Read the model definition and answer for the solid it produces. Units are mm, in the model's axes. Face numbers are marked on the shaded views. A direction names the side the tool comes from. Coordinates: 2 decimals unless noted, no trailing zeros. Order: outer loops, then holes, each group sorted by start corner. A loop starts at its lowest first (then second) coordinate and runs counter-clockwise, first axis right, second up. Notation, with made-up numbers: (-12, 9.5) -> (-8, 9.5) arc R24 ccw to (-8, 35.5) -> close; hole circle Ø10 at (-31.5, 14). An arc over 180 degrees is marked (long way). Use CSV: the item, a comma, the result in double quotes.
```python
from build123d import *

# Parameters (mm, degrees)
F1_DEPTH = 25.4
F2_DEPTH = 25.654


with BuildPart() as f1:
    # F0 (on Front) → F1 (new body)
    with BuildSketch(Plane.XZ):
        with BuildLine():
            ThreePointArc((-15.060614174, 41.9682624685), (-0.0688082783, 50.3511332937), (14.987647146, 42.0849420703))
            ThreePointArc((14.987647146, 42.0849420703), (19.3434405932, 43.5057594661), (23.8204686342, 44.4793500101))
            Line((23.8204686342, 44.4793500101), (1.0321482392, 85.7816260454))
            Line((1.0321482392, 85.7816260454), (-24.0085215463, 44.2917114126))
            ThreePointArc((-24.0085215463, 44.2917114126), (-19.4747765312, 43.3602512097), (-15.060614174, 41.9682624685))
        make_face()
    extrude(amount=-F1_DEPTH)

    # F0 (on Front) → F2 (join)
    with BuildSketch(Plane.XZ):
        with BuildLine():
            Line((-28.8295803882, 36.30369346), (-27.7535005612, 38.0866513657))
            Line((-27.7535005612, 38.0866513657), (-30.7906209519, 44.8054462665))
            ThreePointArc((-30.7906209519, 44.8054462665), (-29.6489661187, 40.624103652), (-29.2771657497, 36.3056819144))
            Line((-29.2771657497, 36.3056819144), (-28.8295803882, 36.30369346))
        make_face()
        Polygon((-30.7906209519, 44.8054462665), (-27.7535005612, 38.0866513657), (-25.0648295944, 42.54151339), align=None)
        with BuildLine():
            Line((-53.3023555948, 36.4124168488), (-30.7906209519, 36.3124056299))
            Line((-30.7906209519, 36.3124056299), (-30.7906209519, 44.8054462665))
            ThreePointArc((-30.7906209519, 44.8054462665), (-62.5500321621, 31.6953988364), (-75.8140902377, 0))
            Line((-75.8140902377, 0), (-75.2328084137, -0.0011871857))
            ThreePointArc((-75.2328084137, -0.0011871857), (-73.1076200485, 9.3092127471), (-67.2269157832, 16.8336588954))
            ThreePointArc((-67.2269157832, 16.8336588954), (-60.6978163865, 20.5368755433), (-53.3023555948, 21.8214424558))
            Line((-53.3023555948, 21.8214424558), (-53.3023555948, 36.4124168488))
        make_face()
        with BuildLine():
            Line((-30.7906209519, 44.8054462665), (-30.7906209519, 36.3124056299))
            Line((-30.7906209519, 36.3124056299), (-29.2771657497, 36.3056819144))
            ThreePointArc((-29.2771657497, 36.3056819144), (-29.6489661187, 40.624103652), (-30.7906209519, 44.8054462665))
        make_face()
        with BuildLine():
            Line((-25.0648295944, 42.54151339), (-16.4788366985, 39.1466793172))
            ThreePointArc((-16.4788366985, 39.1466793172), (-15.832705808, 40.5891269445), (-15.060614174, 41.9682624685))
            ThreePointArc((-15.060614174, 41.9682624685), (-19.4747765312, 43.3602512097), (-24.0085215463, 44.2917114126))
            Line((-24.0085215463, 44.2917114126), (-25.0648295944, 42.54151339))
        make_face()
        with BuildLine():
            ThreePointArc((23.8204686342, 44.4793500101), (19.3434405932, 43.5057594661), (14.987647146, 42.0849420703))
            ThreePointArc((14.987647146, 42.0849420703), (15.7885662341, 40.6763432088), (16.4574657961, 39.2004721052))
            Line((16.4574657961, 39.2004721052), (24.8784135948, 42.5618969449))
            Line((24.8784135948, 42.5618969449), (23.8204686342, 44.4793500101))
        make_face()
        with BuildLine():
            ThreePointArc((-15.060614174, 41.9682624685), (-0.0688082783, 50.3511332937), (14.987647146, 42.0849420703))
            ThreePointArc((14.987647146, 42.0849420703), (19.3434405932, 43.5057594661), (23.8204686342, 44.4793500101))
            Line((23.8204686342, 44.4793500101), (1.0321482392, 85.7816260454))
            Line((1.0321482392, 85.7816260454), (-24.0085215463, 44.2917114126))
            ThreePointArc((-24.0085215463, 44.2917114126), (-19.4747765312, 43.3602512097), (-15.060614174, 41.9682624685))
        make_face()
        with BuildLine():
            ThreePointArc((-24.0085215463, 44.2917114126), (-27.3898564846, 44.6768288461), (-30.7906209519, 44.8054462665))
            Line((-30.7906209519, 44.8054462665), (-25.0648295944, 42.54151339))
            Line((-25.0648295944, 42.54151339), (-24.0085215463, 44.2917114126))
        make_face()
        with BuildLine():
            Line((29.4191831059, 36.0449159855), (31.1962604648, 36.0370210954))
            Line((31.1962604648, 36.0370210954), (31.1962604648, 45.083818219))
            ThreePointArc((31.1962604648, 45.083818219), (29.8777965479, 40.6488917918), (29.4191831059, 36.0449159855))
        make_face()
        with BuildLine():
            Line((31.1962604648, 45.083818219), (31.1962604648, 36.0370210954))
            Line((31.1962604648, 36.0370210954), (53.8473990671, 35.9363905568))
            Line((53.8473990671, 35.9363905568), (53.8473990671, 21.9238056105))
            ThreePointArc((53.8473990671, 21.9238056105), (61.6802350926, 20.4952804957), (68.5044998261, 16.3936448398))
            ThreePointArc((68.5044998261, 16.3936448398), (74.0656549864, 8.8761377727), (76.0360198852, -0.2648152075))
            ThreePointArc((76.0360198852, -0.2648152075), (76.036008316, -0.2874737281), (76.0359736084, -0.310132225))
            Line((76.0359736084, -0.310132225), (76.4985376694, -0.3110769465))
            ThreePointArc((76.4985376694, -0.3110769465), (63.2625699929, 31.7823320468), (31.1962604648, 45.083818219))
        make_face()
        Polygon((24.8784135948, 42.5618969449), (27.686077002, 37.4731985658), (31.1962604648, 45.083818219), align=None)
        with BuildLine():
            Line((31.1962604648, 45.083818219), (27.686077002, 37.4731985658))
            Line((27.686077002, 37.4731985658), (28.4718024235, 36.0491248436))
            Line((28.4718024235, 36.0491248436), (29.4191831059, 36.0449159855))
            ThreePointArc((29.4191831059, 36.0449159855), (29.8777965479, 40.6488917918), (31.1962604648, 45.083818219))
        make_face()
        Polygon((-25.4324655009, -43.1239806736), (-27.9238592306, -38.808760152), (-30.7906209519, -45.2425532036), align=None)
        with BuildLine():
            Line((-30.7906209519, -45.2425532036), (-27.9238592306, -38.808760152))
            Line((-27.9238592306, -38.808760152), (-29.1769886883, -36.6382762629))
            Line((-29.1769886883, -36.6382762629), (-29.2232528573, -36.6383886578))
            ThreePointArc((-29.2232528573, -36.6383886578), (-29.6130237377, -41.012227686), (-30.7906209519, -45.2425532036))
        make_face()
        with BuildLine():
            ThreePointArc((31.1962604648, 45.083818219), (27.4960007799, 44.9324482787), (23.8204686342, 44.4793500101))
            Line((23.8204686342, 44.4793500101), (24.8784135948, 42.5618969449))
            Line((24.8784135948, 42.5618969449), (31.1962604648, 45.083818219))
        make_face()
        with BuildLine():
            Line((-75.2328164085, -0.0028216264), (-75.8140902377, 0))
            ThreePointArc((-75.8140902377, 0), (-62.704573257, -31.9779646787), (-30.7906209519, -45.2425532036))
            Line((-30.7906209519, -45.2425532036), (-30.7906209519, -36.6421964468))
            Line((-30.7906209519, -36.6421964468), (-53.3023555948, -36.6968868137))
            Line((-53.3023555948, -36.6968868137), (-53.3023555948, -22.0399959243))
            ThreePointArc((-53.3023555948, -22.0399959243), (-60.6978163865, -20.7554290119), (-67.2269157832, -17.052212364))
            ThreePointArc((-67.2269157832, -17.052212364), (-73.1534528918, -9.4307777023), (-75.2328164085, -0.0028216264))
        make_face()
        with BuildLine():
            Line((-75.2328084137, -0.0011871857), (-75.8140902377, 0))
            Line((-75.8140902377, 0), (-75.2328164085, -0.0028216264))
            ThreePointArc((-75.2328164085, -0.0028216264), (-75.2328124264, -0.002004406), (-75.2328084137, -0.0011871857))
        make_face()
        with BuildLine():
            Line((-25.4324655009, -43.1239806736), (-30.7906209519, -45.2425532036))
            ThreePointArc((-30.7906209519, -45.2425532036), (-27.6209328908, -45.1308416505), (-24.4669738087, -44.7962613387))
            Line((-24.4669738087, -44.7962613387), (-25.4324655009, -43.1239806736))
        make_face()
        with BuildLine():
            Line((-30.7906209519, -36.6421964468), (-30.7906209519, -45.2425532036))
            ThreePointArc((-30.7906209519, -45.2425532036), (-29.6130237377, -41.012227686), (-29.2232528573, -36.6383886578))
            Line((-29.2232528573, -36.6383886578), (-30.7906209519, -36.6421964468))
        make_face()
        with BuildLine():
            Line((-16.7719402399, -39.6996770897), (-25.4324655009, -43.1239806736))
            Line((-25.4324655009, -43.1239806736), (-24.4669738087, -44.7962613387))
            ThreePointArc((-24.4669738087, -44.7962613387), (-19.855090202, -43.8943444673), (-15.3623330745, -42.5166442684))
            ThreePointArc((-15.3623330745, -42.5166442684), (-16.1287540245, -41.1389939394), (-16.7719402399, -39.6996770897))
        make_face()
        with BuildLine():
            ThreePointArc((24.3490687404, -45.0004789074), (19.7574141393, -44.0529882803), (15.2882742932, -42.6360128042))
            ThreePointArc((15.2882742932, -42.6360128042), (-0.070238078, -51.1034201303), (-15.3623330745, -42.5166442684))
            ThreePointArc((-15.3623330745, -42.5166442684), (-19.855090202, -43.8943444673), (-24.4669738087, -44.7962613387))
            Line((-24.4669738087, -44.7962613387), (0, -87.1743030828))
            Line((0, -87.1743030828), (24.3490687404, -45.0004789074))
        make_face()
        with BuildLine():
            ThreePointArc((16.7501892204, -39.754426672), (16.0838947627, -41.2280252172), (15.2882742932, -42.6360128042))
            ThreePointArc((15.2882742932, -42.6360128042), (19.7574141393, -44.0529882803), (24.3490687404, -45.0004789074))
            Line((24.3490687404, -45.0004789074), (25.387333514, -43.2021515679))
            Line((25.387333514, -43.2021515679), (16.7501892204, -39.754426672))
        make_face()
        with BuildLine():
            Line((29.2589523384, -36.4963110564), (28.047162827, -38.5951920583))
            Line((28.047162827, -38.5951920583), (31.1962604648, -45.5209251562))
            ThreePointArc((31.1962604648, -45.5209251562), (29.8905818384, -41.0917228659), (29.4425640224, -36.4958649872))
            Line((29.4425640224, -36.4958649872), (29.2589523384, -36.4963110564))
        make_face()
        Polygon((31.1962604648, -45.5209251562), (28.047162827, -38.5951920583), (25.387333514, -43.2021515679), align=None)
        with BuildLine():
            ThreePointArc((68.5044998261, -16.9232752549), (61.6802350926, -21.0249109107), (53.8473990671, -22.4534360256))
            Line((53.8473990671, -22.4534360256), (53.8473990671, -36.436575492))
            Line((53.8473990671, -36.436575492), (31.1962604648, -36.4916045291))
            Line((31.1962604648, -36.4916045291), (31.1962604648, -45.5209251562))
            ThreePointArc((31.1962604648, -45.5209251562), (63.1971459801, -32.2848629967), (76.4985376694, -0.3110769465))
            Line((76.4985376694, -0.3110769465), (76.0359736084, -0.310132225))
            ThreePointArc((76.0359736084, -0.310132225), (74.056309909, -9.4264098499), (68.5044998261, -16.9232752549))
        make_face()
        with BuildLine():
            Line((25.387333514, -43.2021515679), (24.3490687404, -45.0004789074))
            ThreePointArc((24.3490687404, -45.0004789074), (27.7627892326, -45.3906262107), (31.1962604648, -45.5209251562))
            Line((31.1962604648, -45.5209251562), (25.387333514, -43.2021515679))
        make_face()
        with BuildLine():
            ThreePointArc((29.4425640224, -36.4958649872), (29.8905818384, -41.0917228659), (31.1962604648, -45.5209251562))
            Line((31.1962604648, -45.5209251562), (31.1962604648, -36.4916045291))
            Line((31.1962604648, -36.4916045291), (29.4425640224, -36.4958649872))
        make_face()
    extrude(amount=-F2_DEPTH)


solid = f1.part
```
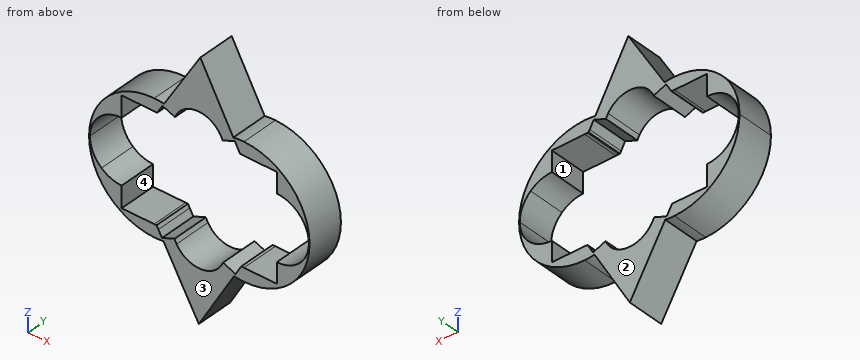
Item 1: Find section A-A, the plane z = -26. Give the vertices of the cut face in (x, y), then the cut area to 3 significant figures.
Return value:
outline,"(-67.7, 0) -> (-53.3, 0) -> (-53.3, 25.65) -> (-67.7, 25.65) -> close; (53.85, 0) -> (68.45, 0) -> (68.45, 25.65) -> (53.85, 25.65) -> close"
area,"744 mm^2"
Item 2: Find section B-B, the plane x = 11. Give the vertices of the cut face in (y, z), then the cut area to 3 significant figures.
Return value:
outline,"(0, -68.12) -> (25.65, -68.12) -> (25.65, -47.36) -> (0, -47.36) -> close; (0, 46.52) -> (25.65, 46.52) -> (25.65, 67.72) -> (0, 67.72) -> close"
area,"1,080 mm^2"
Item 3: Straight lines are drawn through the part: line 1 along Z through (x, y) = (27, 10); line 2 along Z through (x, y) = (-29, 14.5); line 3 along X through (y, z) = (16.5, -17). For each, find the intervals that lie inside material, in ascending order.
Return value:
line 1,"z = -45.33 to -40.41, 38.72 to 44.89"
line 2,"z = -45.21 to -36.94, 36.3 to 44.77"
line 3,"x = -72.57 to -67.29, 68.42 to 73.28"
Item 4: Find section C-C, the plane z = -54.5. Give the vertices of the cut face in (x, y), then the cut area to 3 significant figures.
Return value:
outline,"(-18.86, 0) -> (18.86, 0) -> (18.86, 25.65) -> (-18.86, 25.65) -> close"
area,"968 mm^2"
Item 5: Each of these flat-tipped pins is pushed along its axis until it touches: P1, Ø6, axis at x = -58, y = 7, coming from the -Z side; P2, Ø11.5, axis at y = 7, z = -31.5, coming from the +X side; P3, Ø4, axis at x = 56, y = 5.5, coming from the -Z side. Where does it stop, or does it pass through?
Return value:
P1,"stops at z = -38.18"
P2,"stops at x = 68.62"
P3,"stops at z = -39.36"
Item 6: The mould has two halves that part along X. Classify the marked faces 1 and 2: +X half, -X half, draft (parallel to the pull), parting line (faces both ways), or undercut.
Return value:
face 1,"undercut"
face 2,"draft"
Item 7: A tool of negligible diameter and unlimited length cuts with its end or side. For the marked faces 3 and 4, from which of +Z, -Z, +X, -X, +Y, -Y can it reach the whole face along a straight path? Write none if from no direction.
Return value:
face 3,"+Z, -Z, +X, -X, -Y"
face 4,"+Y, -Y"
